```python
from build123d import *

# Parameters (mm, degrees)
SKETCH4_W           = 40
SKETCH4_H           = 20
BOSS_EXTRUDE2_DEPTH = 2
SKETCH5_R           = 1.25
CUT_EXTRUDE1_DEPTH  = 23.449944321
BOSS_EXTRUDE3_DEPTH = 2.3
SKETCH7_R           = 7.25
BOSS_EXTRUDE4_DEPTH = 1.2
CUT_EXTRUDE2_DEPTH  = 0.2


with BuildPart() as part:
    # Sketch4 → Boss-Extrude2 (new body)
    with BuildSketch(Plane(origin=(0, 0, 0), x_dir=(1, 0, 0), z_dir=(0, 1, 0))):
        Rectangle(SKETCH4_W, SKETCH4_H)
    extrude(amount=BOSS_EXTRUDE2_DEPTH)

    # Sketch5 → Cut-Extrude1 (cut, through all)
    with BuildSketch(Plane(origin=(0, 2, 0), x_dir=(1, 0, 0), z_dir=(0, 1, 0))):
        with Locations(Location((-18.3, 8.3, 0), (0, 0, 270))):
            Circle(SKETCH5_R)
        with Locations(Location((18.3, 8.3, 0), (0, 0, 270))):
            Circle(SKETCH5_R)
        with Locations(Location((-18.3, -8.3, 0), (0, 0, 270))):
            Circle(SKETCH5_R)
        with Locations(Location((18.3, -8.3, 0), (0, 0, 270))):
            Circle(SKETCH5_R)
    extrude(amount=-CUT_EXTRUDE1_DEPTH, mode=Mode.SUBTRACT)

    # Sketch6 → Boss-Extrude3 (add)
    with BuildSketch(Plane.XZ):
        with BuildLine():
            Line((-10.1, 8.65), (10.1, 8.65))
            ThreePointArc((10.1, 8.65), (18.75, 0), (10.1, -8.65))
            Line((10.1, -8.65), (-10.1, -8.65))
            ThreePointArc((-10.1, -8.65), (-18.75, 0), (-10.1, 8.65))
        make_face()
    extrude(amount=BOSS_EXTRUDE3_DEPTH)

    # Sketch7 → Boss-Extrude4 (add)
    with BuildSketch(Plane.XZ.offset(2.3)):
        with Locations(Location((0, 0, 0), (0, 0, 270))):
            Circle(SKETCH7_R)
    extrude(amount=BOSS_EXTRUDE4_DEPTH)

    # Sketch8 → Cut-Extrude2 (cut)
    with BuildSketch(Plane(origin=(0, 2, 0), x_dir=(1, 0, 0), z_dir=(0, 1, 0))):
        with BuildLine():
            Line((-10.706568747, 8.336924947), (10.706568747, 8.336924947))
            ThreePointArc((10.706568747, 8.336924947), (19.043493695, 0), (10.706568747, -8.336924947))
            Line((10.706568747, -8.336924947), (-10.706568747, -8.336924947))
            ThreePointArc((-10.706568747, -8.336924947), (-19.043493695, 0), (-10.706568747, 8.336924947))
        make_face()
    extrude(amount=-CUT_EXTRUDE2_DEPTH, mode=Mode.SUBTRACT)


solid = part.part
```
The listing builds one solid part. Answer for the finished solid, in the listing's coordinates (mm). A direction names the side the tool comes from. Coordinates: 2 decimals unless noted, no trailing zeros. Write each loop counter-clockwise with the first axis right and the second up, starting at its lowest first coordinate (ties: lowest second). Pieces come first, ordered by that corner, then holes. Notation, with made-up numbers: M -7.75,34 L 43.25,34 A21 ccw 43.25,65 Z; hole C -15,27 d8. An arc over 180 degrees is marked long. Use a Markdown table: item, result. Add a question column.
1. Section A-A (y = 0.95) is taken. Give the vertices of the cut face in (x, z), plus the area to 3 significant figures.
2. Section C-C (z = 0) is taken. Give the vertices of the cut face in (x, y).
3. Section D-D (x = 18.3) is taken. Give the vertices of the cut face in (y, z), plus the area to 3 significant figures.
4. Section B-B (x = 8) is taken. Give the vertices of the cut face in (y, z), plus the area to 3 significant figures.
5. Which of the six approach directions +Z, -Z, +X, -X, +Y, -Y give full straight-line access (tool end or side, diameter ignored) to faces 1 (the flat face through (0, -1, 8.65)), 2 (the flat face through (0, 1.8, 0)), 3 (the flat face through (0, 1, 10)), 4 (the cylindrical face through (-17.06, 1.01, 8.14)), 5 (the flat face through (0, -1, -8.65))?
6. For a pull along X with two mould halves and no side action, classify faces 6 (the cylindrical face through (18.748, -1.134, 0.19)), 7 (the flat face through (0, 0, 9)), 8 (the cylindrical face through (17.08, 1.01, 8.03)), 9 (the cylindrical face through (-2.777, -2.892, -6.697)) as +X half, -X half, draft (parallel to the pull), parting line (faces both ways), or undercut.
7. Given P1, Ø3, axis at x = 18.3, z = 8.3, coming from the -Y side; P2, Ø1.8, axis at x = 3.5, y = -1.5, coming from the -Z side; P3, Ø1, axis at x = 3.5, y = -2.5, coming from the +Z side, each flat-ended and moving along its own axis, determine where each tip first touches the part or whether it passes through.
8. Straight lines are drawn through the part: line 1 along X through (y, z) = (0.8, 8.3); line 2 along Z through (x, y) = (-2.5, -0.5); line 3 along Y through (x, z) = (12, -7). For each, find the intervals that lie inside material, in ascending order. Write a range as [from, to].
Data:
| question | item | result |
|---|---|---|
| 1 | outline | M -20,-10 L 20,-10 L 20,10 L -20,10 Z; hole C -18.3,-8.3 d2.5; hole C -18.3,8.3 d2.5; hole C 18.3,-8.3 d2.5; hole C 18.3,8.3 d2.5 |
| 1 | area | 780 mm2 |
| 2 | outline | M -20,0 L -18.75,0 L -18.75,-2.3 L -7.25,-2.3 L -7.25,-3.5 L 7.25,-3.5 L 7.25,-2.3 L 18.75,-2.3 L 18.75,0 L 20,0 L 20,2 L 19.04,2 L 19.04,1.8 L -19.04,1.8 L -19.04,2 L -20,2 Z |
| 3 | outline | M -2.3,-2.75 L 0,-2.75 L 0,-7.05 L 2,-7.05 L 2,-3.44 L 1.8,-3.44 L 1.8,3.44 L 2,3.44 L 2,7.05 L 0,7.05 L 0,2.75 L -2.3,2.75 Z; M 0,-10 L 2,-10 L 2,-9.55 L 0,-9.55 Z; M 0,9.55 L 2,9.55 L 2,10 L 0,10 Z |
| 3 | area | 41.3 mm2 |
| 4 | outline | M -2.3,-8.65 L 0,-8.65 L 0,-10 L 2,-10 L 2,-8.34 L 1.8,-8.34 L 1.8,8.34 L 2,8.34 L 2,10 L 0,10 L 0,8.65 L -2.3,8.65 Z |
| 4 | area | 76.5 mm2 |
| 5 | face 1 | +Z, +X, -X, -Y |
| 5 | face 2 | +Y |
| 5 | face 3 | +Z, +X, -X, +Y, -Y |
| 5 | face 4 | +Y, -Y |
| 5 | face 5 | -Z, +X, -X, -Y |
| 6 | face 6 | +X half |
| 6 | face 7 | draft |
| 6 | face 8 | undercut |
| 6 | face 9 | parting line |
| 7 | P1 | stops at y = 0 |
| 7 | P2 | stops at z = -8.65 |
| 7 | P3 | stops at z = 8.65 |
| 8 | line 1 | x = [-20, -19.55], [-17.05, 17.05], [19.55, 20] |
| 8 | line 2 | z = [-8.65, 8.65] |
| 8 | line 3 | y = [-2.3, 1.8] |
